Can you work these out from the model? Positions are in its coordinate system, mm. Face numbers are marked on the shaded views. A direction names the side the tool comes from. Give positions to 0.01 mm unless a question says otherwise; leave off trailing zeros. Order: outer loops, then holes, each group sorted by start corner. A loop starts at its lowest first (then second) coordinate and runs counter-clockwise, first axis right, second up. Notation, with made-up numbers: (19.5, 34) - (42.5, 34) arc R14 cw to (42.5, 51) - close; hole circle Ø10 at (-29.5, -23). An arc over 180 degrees is marked (long way). Return JSON: item names as keys, results as strings.
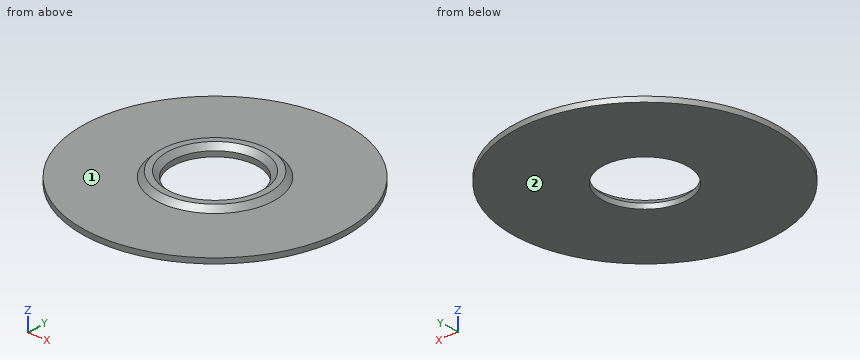
```python
from build123d import *

# Parameters (mm, degrees)
SZKIC1_R                    = 25
SZKIC1_R_2                  = 8.1
DODANIE_WYCI_GNI_CIE1_DEPTH = 1
SZKIC2_R                    = 11.3
SZKIC2_R_2                  = 8.1
DODANIE_WYCI_GNI_CIE2_DEPTH = 1
DODANIE_WYCI_GNI_CIE2_TAPER = 45


with BuildPart() as part:
    # Szkic1 → Dodanie-wyciągnięcie1 (new body)
    with BuildSketch(Plane.XY):
        with Locations((-0.065846009, 4.978571429)):
            Circle(SZKIC1_R)
        with Locations((-0.065846009, 4.978571429)):
            Circle(SZKIC1_R_2, mode=Mode.SUBTRACT)
    extrude(amount=-DODANIE_WYCI_GNI_CIE1_DEPTH)

    # Szkic2 → Dodanie-wyciągnięcie2 (add)
    with BuildSketch(Plane.XY):
        with Locations((-0.065846009, 4.978571429)):
            Circle(SZKIC2_R)
        with Locations((-0.065846009, 4.978571429)):
            Circle(SZKIC2_R_2, mode=Mode.SUBTRACT)
    extrude(amount=DODANIE_WYCI_GNI_CIE2_DEPTH, taper=DODANIE_WYCI_GNI_CIE2_TAPER)


solid = part.part
```
1. If I drill on L1, parallel to Z at x = -12, y = -15; L2, parallel to Y at x = -3.5, z = -0.6; L3, parallel to Y at x = 14.5, z = -0.1, over which ranges is the centre line in solid material (lowest first)? Write a range as [from, to].
Checks:
{"L1": "[-1, 0]", "L2": "[-19.78, -2.36], [12.31, 29.74]", "L3": "[-15.34, 25.3]"}
2. Suppose I cut it at B-B (x = 22.5). List the corners of the cut face in (y, z) for me.
Checks:
{"outline": "(-5.78, -1) - (15.74, -1) - (15.74, 0) - (-5.78, 0) - close"}
3. Suppose I cut it at C-C (y = 17.5). List the corners of the cut face in (x, z) for me.
Checks:
{"outline": "(-21.7, -1) - (21.57, -1) - (21.57, 0) - (-21.7, 0) - close"}
4. Suppose I cut it at A-A (z = -0.55). List the corners of the cut face in (x, y) for me, plus the area to 3 significant figures.
Checks:
{"outline": "circle Ø50 at (-0.07, 4.98); hole circle Ø16.2 at (-0.07, 4.98)", "area": "1,760 mm^2"}
5. For pin 1 Ø1 at (y, z) = (-11, 0) entering from +X; pin 2 Ø1.5 at (x, y) = (-11, -10.5) entering from +Z, each with a flat end and sliding along its axis, tell me the tip position at first contact or that it passes through.
Checks:
{"pin 1": "x = 19.57", "pin 2": "z = 0"}
6. On a 3-axis mill with a long thin cutter (end or side, diameter ignored), from which of +Z, -Z, +X, -X, +Y, -Y can I reach the whole of each face in a straight line? I mean the marked faces 1 and 2. Say none if no direction works.
Checks:
{"face 1": "+Z", "face 2": "-Z, +X, -X, +Y, -Y"}
